The listing builds one solid part. Answer for the finished solid, in the listing's coordinates (mm). A direction names the side the tool comes from. Give positions to 0.01 mm unless a question says otherwise; leave off trailing zeros. Write each loop counter-clockwise with the first axis right and the second up, starting at its lowest first coordinate (ties: lowest second). Pieces come first, ordered by that corner, then holes. Notation, with made-up numbers: M 11,83.5 L 32,83.5 A24 cw 32,95.5 Z; hole C -3,17 d8. An arc over 180 degrees is marked long. Return JSON: item names as keys, results as strings.
from build123d import *

# Parameters (mm, degrees)
SKETCH_1_W          = 200
SKETCH_1_H          = 200
SKETCH_1_W_2        = 51
SKETCH_1_H_2        = 51
EXTRUDE_1_DEPTH     = 20
SKETCH_1_2_W        = 200
SKETCH_1_2_H        = 200
EXTRUDE_2_DEPTH     = 5
SKETCH_2_W          = 200
SKETCH_2_H          = 200
SKETCH_2_W_2        = 190
SKETCH_2_H_2        = 190
CUT_EXTRUDE_1_DEPTH = 10
FILLET_1_R          = 10


with BuildPart() as part:
    # 草图1 → 凸台-拉伸1 (new body)
    with BuildSketch(Plane(origin=(0, 0, 0), x_dir=(1, 0, 0), z_dir=(0, 1, 0))):
        Rectangle(SKETCH_1_W, SKETCH_1_H)
        with Locations((0, 60)):
            Rectangle(SKETCH_1_W_2, SKETCH_1_H_2, mode=Mode.SUBTRACT)
        with Locations((-60, 60)):
            Rectangle(SKETCH_1_W_2, SKETCH_1_H_2, mode=Mode.SUBTRACT)
        with Locations((60, 60)):
            Rectangle(SKETCH_1_W_2, SKETCH_1_H_2, mode=Mode.SUBTRACT)
        Rectangle(SKETCH_1_W_2, SKETCH_1_H_2, mode=Mode.SUBTRACT)
        with Locations((60, 0)):
            Rectangle(SKETCH_1_W_2, SKETCH_1_H_2, mode=Mode.SUBTRACT)
        with Locations((0, -60)):
            Rectangle(SKETCH_1_W_2, SKETCH_1_H_2, mode=Mode.SUBTRACT)
        with Locations((60, -60)):
            Rectangle(SKETCH_1_W_2, SKETCH_1_H_2, mode=Mode.SUBTRACT)
        with Locations((-60, 0)):
            Rectangle(SKETCH_1_W_2, SKETCH_1_H_2, mode=Mode.SUBTRACT)
        with Locations((-60, -60)):
            Rectangle(SKETCH_1_W_2, SKETCH_1_H_2, mode=Mode.SUBTRACT)
    extrude(amount=EXTRUDE_1_DEPTH)

    # 草图1<2> → 凸台-拉伸2 (add)
    with BuildSketch(Plane(origin=(0, 0, 0), x_dir=(1, 0, 0), z_dir=(0, 1, 0))):
        Rectangle(SKETCH_1_2_W, SKETCH_1_2_H)
    extrude(amount=EXTRUDE_2_DEPTH)

    # 草图2 → 切除-拉伸1 (cut)
    with BuildSketch(Plane(origin=(0, 20, 0), x_dir=(1, 0, 0), z_dir=(0, 1, 0))):
        Rectangle(SKETCH_2_W, SKETCH_2_H)
        Rectangle(SKETCH_2_W_2, SKETCH_2_H_2, mode=Mode.SUBTRACT)
    extrude(amount=-CUT_EXTRUDE_1_DEPTH, mode=Mode.SUBTRACT)

    # 圆角1
    fillet_1_edges = [part.edges().sort_by_distance(p)[0] for p in [
        (-100, 5, 100),
        (100, 5, 100),
        (-100, 5, -100),
        (100, 5, -100),
        (-95, 15, -95),
        (95, 15, -95),
        (95, 15, 95),
        (-95, 15, 95),
    ]]
    fillet(fillet_1_edges, radius=FILLET_1_R)


solid = part.part
Item 1: Which of the six approach directions +Z, -Z, +X, -X, +Y, -Y give full straight-line access (tool end or side, diameter ignored) to faces 4 (the flat face through (60, 5, 60)), 5 (the flat face through (-1, 0, -1)), 6 (the flat face through (-95, 15, 1))?
Geometry results:
{"face 4": "+Y", "face 5": "+Z, -Z, +X, -X, -Y", "face 6": "+Z, -Z, -X, +Y"}
Item 2: A cutting plane is placed at C-C, the plane y = 13. Count the separate pieces of the cut face and the enclosed holes in it, plus the area to 3 significant figures.
Geometry results:
{"separate pieces": "1", "enclosed holes": "9", "area": "12,600 mm2"}
Item 3: Determine the mould class of faces 1 (the cylindrical face through (92.15, 14.93, -91.99)), 2 (the cylindrical face through (96.99, 5.07, 97.15)), 3 (the flat face through (-85.5, 12, -60)) for opening direction Z: +Z half, -Z half, draft (parallel to the pull), parting line (faces both ways), or undercut.
Geometry results:
{"face 1": "-Z half", "face 2": "+Z half", "face 3": "undercut"}
Item 4: Given pin 1 Ø12 at (x, y) = (-36.5, 16.5) entering from +Z; pin 2 Ø15.5 at (x, z) = (-49.5, 47.5) entering from +Y; pin 3 Ø8 at (y, z) = (15, -33) entering from +X, each flat-ended and moving along its own axis, determine where each tip first touches the part or whether it passes through.
Geometry results:
{"pin 1": "stops at z = 95", "pin 2": "stops at y = 5", "pin 3": "stops at x = 95"}
Item 5: Find the intervals of material crossed by line 1 (X direction, y = 9.25, z = -80.5); line 2 (Z direction, x = 37, y = 17), in increasing order.
Geometry results:
{"line 1": "x = -100 to -85.5, -34.5 to -25.5, 25.5 to 34.5, 85.5 to 100", "line 2": "z = -95 to -85.5, -34.5 to -25.5, 25.5 to 34.5, 85.5 to 95"}
Item 6: A cutting plane is placed at D-D, the plane z = -62. Write down the section's boundary in (x, y).
Geometry results:
{"outline": "M -100,0 L 100,0 L 100,10 L 95,10 L 95,20 L 85.5,20 L 85.5,5 L 34.5,5 L 34.5,20 L 25.5,20 L 25.5,5 L -25.5,5 L -25.5,20 L -34.5,20 L -34.5,5 L -85.5,5 L -85.5,20 L -95,20 L -95,10 L -100,10 Z"}
Item 7: A cutting plane is placed at B-B, the plane x = 40.5. Write down the section's boundary in (y, z), plus the area to 4 significant figures.
Geometry results:
{"outline": "M 0,-100 L 10,-100 L 10,-95 L 20,-95 L 20,-85.5 L 5,-85.5 L 5,-34.5 L 20,-34.5 L 20,-25.5 L 5,-25.5 L 5,25.5 L 20,25.5 L 20,34.5 L 5,34.5 L 5,85.5 L 20,85.5 L 20,95 L 10,95 L 10,100 L 0,100 Z", "area": "1,605 mm2"}
Item 8: A cutting plane is placed at A-A, the plane z = -30. Write down the section's boundary in (x, y).
Geometry results:
{"outline": "M -100,0 L 100,0 L 100,10 L 95,10 L 95,20 L -95,20 L -95,10 L -100,10 Z"}
